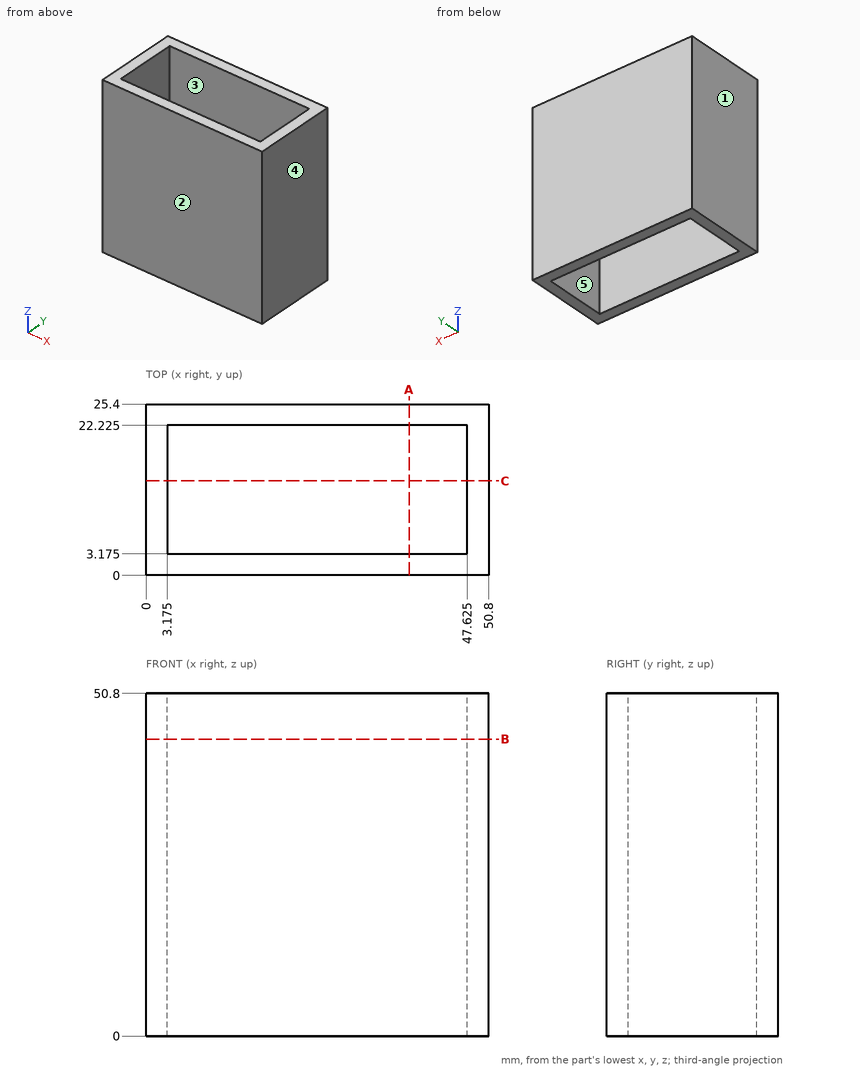
Drawing for the job (mm, zero at the part's lowest x, y, z). A direction names the side the tool comes from. Coordinates: 2 decimals unless noted, no trailing zeros. Order: outer loops, then holes, each group sorted by start corner. A loop starts at its lowest first (then second) coordinate and runs counter-clockwise, first axis right, second up. Notation, with made-up numbers: (13.25, -16.5) - (32.25, -16.5) arc R15 cw to (32.25, -1.5) - close; hole circle Ø3 at (75, 12). An arc over 180 degrees is marked (long way). Use a Markdown table: item, result. Add a question column.
(1) Pull direction X, two halves, no side cores. Call the marked faces 1, 2 and 3: +X half, -X half, draft (parallel to the pull), parting line (faces both ways), or undercut.
(2) Drill centre lines: line 1 along X through (y, z) = (19.25, 41.5) (3 decimals); line 2 along Y through (x, z) = (17, 24) (3 decimals). Where is each one in solid material? Low to high. Write a range as [from, to].
(3) Saw through at A-A (x = 39). Give the cut face in (y, z) (3 decimals), then the cut area to 3 significant figures.
(4) Saw through at B-B (z = 44). Give the cut face in (x, y) (3 decimals).
(5) Saw through at C-C (y = 14). Give the cut face in (x, z) (3 decimals), then the cut area to 3 significant figures.
(6) Which spindle directions (+Z, -Z, +X, -X, +Y, -Y) get a long thin tool onto all of the face, cutting with end or side? Do the marked faces 4 and 5. Say none if no direction does.
Solved:
| question | item | result |
|---|---|---|
| 1 | face 1 | -X half |
| 1 | face 2 | draft |
| 1 | face 3 | undercut |
| 2 | line 1 | x = [0, 3.175], [47.625, 50.8] |
| 2 | line 2 | y = [0, 3.175], [22.225, 25.4] |
| 3 | outline | (0, 0) - (3.175, 0) - (3.175, 50.8) - (0, 50.8) - close; (22.225, 0) - (25.4, 0) - (25.4, 50.8) - (22.225, 50.8) - close |
| 3 | area | 323 mm² |
| 4 | outline | (0, 0) - (50.8, 0) - (50.8, 25.4) - (0, 25.4) - close; hole (3.175, 3.175) - (47.625, 3.175) - (47.625, 22.225) - (3.175, 22.225) - close |
| 5 | outline | (0, 0) - (3.175, 0) - (3.175, 50.8) - (0, 50.8) - close; (47.625, 0) - (50.8, 0) - (50.8, 50.8) - (47.625, 50.8) - close |
| 5 | area | 323 mm² |
| 6 | face 4 | +Z, -Z, +X, +Y, -Y |
| 6 | face 5 | +Z, -Z |
